from build123d import *

# Parameters (mm, degrees)
EXTRUDE_1_DEPTH      = 3
EXTRUDE_1_DEPTH_BACK = 3
SKETCH_1_R           = 2
SKETCH_1_R_2         = 1
SKETCH_2_W           = 130
SKETCH_2_H           = 40
EXTRUDE_2_DEPTH      = 10
SKETCH_3_W           = 41
SKETCH_3_H           = 20
CUT_EXTRUDE_1_DEPTH  = 10
FILLET_1_R           = 10
HOLE_WIZARD_M3_1_D   = 3.4
FILLET_4_R           = 10
SKETCH_6_R           = 2.944419646
EXTRUDE_3_DEPTH      = 1


with BuildPart() as part:
    # 스케치1 → 보스-돌출1 (new, two sides: drawn at the far end of the back side and taken through both)
    with BuildSketch(Plane.XY.offset(-EXTRUDE_1_DEPTH_BACK)):
        with BuildLine():
            Line((0, 20), (45, 20))
            Line((45, 20), (45, -20))
            Line((45, -20), (0, -20))
            ThreePointArc((0, -20), (-20, 0), (0, 20))
        make_face()
        Circle(SKETCH_1_R, mode=Mode.SUBTRACT)
        with Locations((0, 16.16)):
            Circle(SKETCH_1_R_2, mode=Mode.SUBTRACT)
        with Locations((16.16, 0)):
            Circle(SKETCH_1_R_2, mode=Mode.SUBTRACT)
        with Locations((0, -16.16)):
            Circle(SKETCH_1_R_2, mode=Mode.SUBTRACT)
        with Locations((-16.16, 0)):
            Circle(SKETCH_1_R_2, mode=Mode.SUBTRACT)
    extrude(amount=EXTRUDE_1_DEPTH + EXTRUDE_1_DEPTH_BACK)

    # 스케치2 → 보스-돌출2 (add)
    with BuildSketch(Plane(origin=(45, 0, 0), x_dir=(0, 0, -1), z_dir=(1, 0, 0))):
        Rectangle(SKETCH_2_W, SKETCH_2_H)
    extrude(amount=EXTRUDE_2_DEPTH)

    # 스케치3 → 컷-돌출1 (cut)
    with BuildSketch(Plane(origin=(55, 0, 0), x_dir=(0, 0, -1), z_dir=(1, 0, 0))):
        with Locations((32.5, -10)):
            Rectangle(SKETCH_3_W, SKETCH_3_H)
        with Locations((-32.5, -10)):
            Rectangle(SKETCH_3_W, SKETCH_3_H)
    extrude(amount=-CUT_EXTRUDE_1_DEPTH, mode=Mode.SUBTRACT)

    # 필렛1
    fillet_1_edges = [part.edges().sort_by_distance(p)[0] for p in [
        (55, 20, 0),
    ]]
    fillet(fillet_1_edges, radius=FILLET_1_R)

    # M3 여유 구멍1 (through all)
    with Locations(Plane(origin=(55, 0, 0), x_dir=(0, 0, -1), z_dir=(1, 0, 0))):
        with Locations((-57.5, -5.5), (-57.5, -14.5), (-7.2, -5.5), (-7.2, -14.5), (7.2, -5.5), (7.2, -14.5), (57.5, -5.5), (57.5, -14.5)):
            Hole(HOLE_WIZARD_M3_1_D / 2)

    # 필렛4
    fillet_4_edges = [part.edges().sort_by_distance(p)[0] for p in [
        (50, -20, -65),
        (50, -20, 65),
    ]]
    fillet(fillet_4_edges, radius=FILLET_4_R)

    # 스케치6 → 보스-돌출3 (add)
    with BuildSketch(Plane(origin=(55, 0, 0), x_dir=(0, 0, -1), z_dir=(1, 0, 0))):
        with Locations(Location((0, -10, 0), (0, 0, 180))):
            Circle(SKETCH_6_R)
    extrude(amount=EXTRUDE_3_DEPTH)


solid = part.part
Here's how the part is built. I have some questions about the finished solid (model axes, mm). A direction names the side the tool comes from. Round coordinates to 2 decimals unless told otherwise and drop trailing zeros. Loops run counter-clockwise (first coordinate to the right, second up) from the corner with the lowest first, then second, coordinate; pieces in that order, holes last. Notation, with made-up numbers: (-8.75, -26.5) - (19.25, -26.5) arc R22 ccw to (19.25, -8.5) - close; hole circle Ø4 at (81.25, 12.25). An arc over 180 degrees is marked (long way). One line per question, with ' | ' between items. Start each with the question number.
Q1. I want a section at C-C (x = 28). Write out the boundary of the cut face in (y, z), then the cut area to 3 significant figures.
Q2. I want a section at D-D (z = 40.5). Write out the boundary of the cut face in (x, y).
Q3. Please list where these lines run through material, in increasing order: line 1 (Y direction, x = 0, z = -1.4); line 2 (Z direction, x = 50, y = -2); line 3 (X direction, y = 16, z = 0). Write a range as [from, to].
Q4. Will these pins go through, and if not, where does the flat tip stop? pin 1 (8 mm diameter, centred on x = 48, z = -31, fed in from -Y); pin 2 (5.5 mm diameter, centred on y = -14.5, z = -57.5, fed in from -X); pin 3 (10 mm diameter, centred on y = -9.5, z = -21, fed in from -X); pin 4 (4 mm diameter, centred on x = 36.5, y = -8, fed in from -Z).
Q5. We'd pull the mould along Y, two halves only. Please class faces 1 (the cylindrical face through (49.93, -6.15, 8.77)), 2 (the cylindrical face through (50.07, -16.99, -62.15)), 3 (the flat face through (50, -10, 53)), 4 (the cylindrical face through (49.93, -13.99, 8.82)): +Y half, -Y half, draft (parallel to the pull), parting line (faces both ways), or undercut.
Q6. For faces 5 (the cylindrical face through (-20, 0, 0)), 6 (the cylindrical face through (49.93, -14.43, -59.2)), 7 (the flat face through (50, -10, -53)), 8 (the flat face through (45, 5, -34)), 9 (the flat face through (13, 0, 3)), which set-ups out of +Z, -Z, +X, -X, +Y, -Y let a thin tool reach every point of the face, with its end or its side?
Q7. I want a section at A-A (z = -7.2). Write out the boundary of the cut face in (x, y), then the cut area to 3 significant figures.
Q8. I want a section at B-B (y = -5.5). State how many separate pieces and enclosed holes the cut face has, then the cut area to 3 significant figures.
Response values:
1) outline: (-20, -3) - (20, -3) - (20, 3) - (-20, 3) - close | area: 240 mm²
2) outline: (45, 0) - (55, 0) - (55, 10) arc R10 ccw to (45, 20) - close
3) line 1: y = [-20, -17.16], [-15.16, -2], [2, 15.16], [17.16, 20] | line 2: z = [-65, -53], [-12, 12], [53, 65] | line 3: x = [-12, -0.99], [0.99, 53]
4) pin 1: stops at y = 0 | pin 2: stops at x = 45 | pin 3: passes through | pin 4: stops at z = -3
5) face 1: undercut | face 2: -Y half | face 3: draft | face 4: undercut
6) face 5: +Z, -Z, -X | face 6: +X, -X | face 7: +X, -X, -Y | face 8: -Z, -X, +Y, -Y | face 9: +Z, -X, +Y, -Y
7) outline: (45, -20) - (55, -20) - (55, -16.2) - (45, -16.2) - close; (45, -12.8) - (55, -12.8) - (55, -7.2) - (45, -7.2) - close; (45, -3.8) - (55, -3.8) - (55, 10) arc R10 ccw to (45, 20) - close | area: 311 mm²
8) separate pieces: 7 | enclosed holes: 0 | area: 729 mm²
